Solid Edge part; units mm, degrees
sketch "Sketch1" plane through (0, 0, 0) normal (0, 0, 1) x (1, 0, 0)
  circle A0 centre (0, 0) radius 6.4452
extrude "Protrusion1" add sketch "Sketch1" along normal blind 4.7625
sketch "Sketch2" plane through (0, 0, 0) normal (0, 0, -1) x (1, 0, 0)
  circle A0 centre (0, 0) radius 3.175
extrude "Protrusion2" add sketch "Sketch2" along normal blind 25.4
sketch "Sketch3" plane through (0, 0, -25.4) normal (0, 0, -1) x (1, 0, 0)
  circle A0 centre (0, 0) radius 3.1747
extrude "Cutout1" cut sketch "Sketch3" against normal blind 25.3746 flip side to cut
sketch "Sketch4" plane through (0, 0, 4.7625) normal (0, 0, 1) x (1, 0, 0)
  line L0 (-3.2664, 5.5562) -> (3.2664, 5.5562)
extrude "Cutout2" cut sketch "Sketch4" against normal up to next material side at (0, 5.6062, 4.7625)
sketch "Sketch5" plane through (0, 0, 0) normal (1, 0, 0) x (0, 1, 0)
  line L0 (-0.7937, -25.4) -> (-3.1747, -21.276)
revolve "RevolvedCutout1" cut sketch "Sketch5" angle 360 about axis through (0, 0, -14.7796) along (0, 0, 1) material side at (0, -2.0275, -23.363)
pattern_circular "Pattern1" count 6 over 360 about axis through (0, 0, 4.7625) along (0, 0, 1) of "Cutout2"
properties part number "24100261"
Geometry check sheet. Reference: the model listing, model coordinates, mm. A direction names the side the tool comes from. Give positions to 0.01 mm unless a question says otherwise; leave off trailing zeros. Write each loop counter-clockwise with the first axis right and the second up, starting at its lowest first coordinate (ties: lowest second). Pieces come first, ordered by that corner, then holes. Notation, with made-up numbers: (81, -33.75) - (100, -33.75) arc R18 ccw to (100, -7.75) - close; hole circle Ø8 at (31.5, 30.5). An arc over 180 degrees is marked (long way). Put each result on its own line as item: value.
1. Sectioned sample at B-B, the plane z = -10. Enter the section's corners in (x, y), plus the area to 3 significant figures.
Ans:
outline: circle Ø6.35 at (0, 0)
area: 31.7 mm²
2. Sectioned sample at C-C, the plane y = -4.25. Enter the section's corners in (x, z), plus the area to 3 significant figures.
Ans:
outline: (-3.96, 0) - (3.96, 0) - (3.96, 4.76) - (-3.96, 4.76) - close
area: 37.7 mm²
3. Draft check along Z on faces 3 (the cylindrical face through (2.93, 1.22, -10.8)), 4 (the flat face through (0, 0, -25.4)), 5 (the flat face through (0, 0, 4.762)). Enter one of: +Z half, -Z half, draft (parallel to the pull), parting line (faces both ways), or undercut.
Ans:
face 3: draft
face 4: -Z half
face 5: +Z half
4. Sectioned sample at D-D, the plane x = -5.5. Enter the section's corners in (y, z).
Ans:
outline: (-1.59, 0) - (1.59, 0) - (1.59, 4.76) - (-1.59, 4.76) - close
5. Thickness scan on line 1 (Z direction, x = -2.25, y = -2.5); line 2 (Y direction, x = 2.5, z = -13); line 3 (X direction, y = 0, z = -9). Record the ranges inside material, lowest first.
Ans:
line 1: z = 0 to 4.76
line 2: y = -1.96 to 1.96
line 3: x = -3.17 to 3.17
6. Set-up check for faces 1 (the flat face through (3, 3, 0)), 2 (the flat face through (-4.834, 2.739, 2.415)): record each of +Z, -Z, +X, -X, +Y, -Y from which the full face is reachable in a straight line by a thin tool's end or side.
Ans:
face 1: -Z
face 2: +Z, -Z, -X, +Y
7. Go/stop test with flat-tipped pins: pin 1 (5 mm diameter, centred on x = -2, y = 3, fed in from -Z); pin 2 (1.9 mm diameter, centred on x = -1, y = 1.5, fed in from -Z); pin 3 (5 mm diameter, centred on x = -1, z = -11.5, fed in from +Y). Record where each tip stops, or that it passes through.
Ans:
pin 1: stops at z = -24.86
pin 2: stops at z = -25.3
pin 3: stops at y = 3.17
